```python
from build123d import *

# Parameters (mm, degrees)
SKETCH3_R               = 127.8
BOSS_EXTRUDE1_DEPTH     = 22
CUT_EXTRUDE1_DEPTH      = 1
CUT_EXTRUDE1_DEPTH_BACK = 45
SKETCH7_R               = 107
SKETCH7_R_2             = 34.7
CUT_EXTRUDE2_DEPTH      = 2
CHAMFER1_SIZE           = 1.5
CHAMFER2_SIZE           = 1.5
CHAMFER3_SIZE           = 1.5
CHAMFER4_SIZE           = 1.5


with BuildPart() as part:
    # Sketch3 → Boss-Extrude1 (new body, symmetric)
    with BuildSketch(Plane.XY):
        Circle(SKETCH3_R)
    extrude(amount=BOSS_EXTRUDE1_DEPTH, both=True)

    # Sketch6 → Cut-Extrude1 (cut, two sides)
    with BuildSketch(Plane.XY.offset(22)) as cut_extrude1_sk:
        with BuildLine():
            Line((-6, 19.078784028), (-6, 23.3))
            Line((-6, 23.3), (6, 23.3))
            Line((6, 23.3), (6, 19.078784028))
            ThreePointArc((6, 19.078784028), (0, -20), (-6, 19.078784028))
        make_face()
    extrude(amount=CUT_EXTRUDE1_DEPTH, mode=Mode.SUBTRACT)
    extrude(cut_extrude1_sk.sketch, amount=-CUT_EXTRUDE1_DEPTH_BACK, mode=Mode.SUBTRACT)

    # Sketch7 → Cut-Extrude2 (cut)
    with BuildSketch(Plane.XY.offset(22)):
        Circle(SKETCH7_R)
        Circle(SKETCH7_R_2, mode=Mode.SUBTRACT)
    cut_extrude2 = extrude(amount=-CUT_EXTRUDE2_DEPTH, mode=Mode.SUBTRACT)

    # Mirror1: Cut-Extrude2 across plane
    add(cut_extrude2.mirror(Plane.XY), mode=Mode.SUBTRACT)

    # Chamfer1
    chamfer1_edges = [part.edges().sort_by_distance(p)[0] for p in [
        (-107, 0, 20),
    ]]
    chamfer(chamfer1_edges, length=CHAMFER1_SIZE)

    # Chamfer2
    chamfer2_edges = [part.edges().sort_by_distance(p)[0] for p in [
        (-34.7, 0, 20),
    ]]
    chamfer(chamfer2_edges, length=CHAMFER2_SIZE)

    # Chamfer3
    chamfer3_edges = [part.edges().sort_by_distance(p)[0] for p in [
        (0, -20, 22),
    ]]
    chamfer(chamfer3_edges, length=CHAMFER3_SIZE)

    # Chamfer4
    chamfer4_edges = [part.edges().sort_by_distance(p)[0] for p in [
        (0, -20, -22),
        (-107, 0, -20),
        (-34.7, 0, -20),
    ]]
    chamfer(chamfer4_edges, length=CHAMFER4_SIZE)


solid = part.part
```
The model under review builds one solid part; all positions refer to its coordinate system, in mm. A direction names the side the tool comes from. Round coordinates to 2 decimals unless told otherwise and drop trailing zeros. Order: outer loops, then holes, each group sorted by start corner. A loop starts at its lowest first (then second) coordinate and runs counter-clockwise, first axis right, second up.
Item 1: For pin 1 (4 mm diameter, centred on x = 73.5, y = 45.5, fed in from -Z); pin 2 (2 mm diameter, centred on x = -57.5, y = 15, fed in from +Z); pin 3 (4 mm diameter, centred on y = 39, z = -7, fed in from -X), all flat-tipped, find the tip position at first contact; note any pin that passes through.
Working result:
pin 1: stops at z = -20
pin 2: stops at z = 20
pin 3: stops at x = -122.33
Item 2: Add section B-B, the plane z = 16. State the section outline as (x, y) points.
Working result:
outline: circle Ø255.6 at (0, 0); hole (-6, 19.08) arc R20 ccw (long way) to (6, 19.08) - (6, 23.3) - (-6, 23.3) - close
Item 3: Machinability: for faces 1 (the flat face through (15, 16, -22)), 2 (the flat face through (45, 1, 20)), 3 (the flat face through (45, 1, -20)), which of the approach directions +Z, -Z, +X, -X, +Y, -Y give a long, thin tool a straight path to every point of the face, cutting with its end or side? Answer none if there is none.
Working result:
face 1: -Z, +X, -X, +Y, -Y
face 2: +Z
face 3: -Z
Item 4: To check wall thickness, follow probe 1 along Y at (x, z) = (0, -21); probe 2 along Y at (x, z) = (0, -21.8); probe 3 along Y at (x, z) = (0, 12). State the ranges of each line that lie inside material, in increasing order.
Working result:
probe 1: y = -127.8 to -106.5, -35.2 to -20.5, 23.3 to 35.2, 106.5 to 127.8
probe 2: y = -127.8 to -107, -34.7 to -21.3, 23.3 to 34.7, 107 to 127.8
probe 3: y = -127.8 to -20, 23.3 to 127.8
Item 5: Draft analysis for pull direction X (two halves, no side actions). For faces 4 (the flat face through (-29, -104, 22)), 5 (the cylindrical face through (-27.7, -124.76, 0.31)), 6 (the conical face through (0.81, -20.223, 20.74)), state which applies: released by +X, released by -X, zero draft, split by the parting line, or undercut.
Working result:
face 4: zero draft
face 5: split by the parting line
face 6: undercut
